from build123d import *

# Parameters (mm, degrees)
STRUCTURAL_MEMBER1_DEPTH = 900
SKETCH12_R               = 4.7625
CUT_EXTRUDE1_DEPTH       = 454.210052427
CUT_EXTRUDE2_DEPTH       = 40
SKETCH16_R               = 4.7625
CUT_EXTRUDE3_DEPTH       = 454.210052526
SKETCH17_R               = 4.7625
CUT_EXTRUDE4_DEPTH       = 454.210052526


with BuildPart() as part:
    # Sketch11 → Structural Member1 (new body)
    with BuildSketch(Plane(origin=(-450, 0, 0), x_dir=(0, 0, -1), z_dir=(1, 0, 0))):
        with BuildLine():
            Line((0, -38.1), (0, 38.1))
            Line((0, 38.1), (38.0492, 38.1))
            Line((38.0492, 38.1), (38.0492, 35.942335136))
            ThreePointArc((38.0492, 35.942335136), (37.447280466, 34.300554363), (35.926803066, 33.436899509))
            Line((35.926803066, 33.436899509), (12.283671721, 29.496090157))
            ThreePointArc((12.283671721, 29.496090157), (8.178382741, 27.164222052), (6.5532, 22.731413966))
            Line((6.5532, 22.731413966), (6.5532, -22.731413966))
            ThreePointArc((6.5532, -22.731413966), (8.178382741, -27.164222052), (12.283671721, -29.496090157))
            Line((12.283671721, -29.496090157), (35.926803066, -33.436899509))
            ThreePointArc((35.926803066, -33.436899509), (37.447280466, -34.300554363), (38.0492, -35.942335136))
            Line((38.0492, -35.942335136), (38.0492, -38.1))
            Line((38.0492, -38.1), (0, -38.1))
        make_face()
    extrude(amount=STRUCTURAL_MEMBER1_DEPTH)

    # Sketch12 → Cut-Extrude1 (cut, through all)
    with BuildSketch(Plane(origin=(0, 0, 0), x_dir=(1, 0, 0), z_dir=(0, 1, 0))):
        with Locations(Location((-425, 20, 0), (0, 0, 270))):
            Circle(SKETCH12_R)
        with Locations(Location((425, 20, 0), (0, 0, 270))):
            Circle(SKETCH12_R)
    extrude(amount=-CUT_EXTRUDE1_DEPTH, mode=Mode.SUBTRACT)

    # Sketch15 → Cut-Extrude2 (cut)
    with BuildSketch(Plane(origin=(0, 0, -6.5532), x_dir=(-1, 0, 0), z_dir=(0, 0, -1))):
        with BuildLine():
            Line((-412.5, -33.1), (-437.5, -33.1))
            ThreePointArc((-437.5, -33.1), (-442.5, -28.1), (-437.5, -23.1))
            Line((-437.5, -23.1), (-412.5, -23.1))
            ThreePointArc((-412.5, -23.1), (-407.5, -28.1), (-412.5, -33.1))
        make_face()
        with BuildLine():
            Line((412.5, -33.1), (437.5, -33.1))
            ThreePointArc((437.5, -33.1), (442.5, -28.1), (437.5, -23.1))
            Line((437.5, -23.1), (412.5, -23.1))
            ThreePointArc((412.5, -23.1), (407.5, -28.1), (412.5, -33.1))
        make_face()
    extrude(amount=CUT_EXTRUDE2_DEPTH, mode=Mode.SUBTRACT)

    # Sketch16 → Cut-Extrude3 (cut, through all)
    with BuildSketch(Plane(origin=(0, 0, 0), x_dir=(1, 0, 0), z_dir=(0, 1, 0))):
        with Locations(Location((-192.7, 20, 0), (0, 0, 270))):
            Circle(SKETCH16_R)
        with Locations(Location((-157.7, 20, 0), (0, 0, 270))):
            Circle(SKETCH16_R)
        with Locations(Location((157.7, 20, 0), (0, 0, 90))):
            Circle(SKETCH16_R)
        with Locations(Location((192.7, 20, 0), (0, 0, 90))):
            Circle(SKETCH16_R)
    extrude(amount=CUT_EXTRUDE3_DEPTH, mode=Mode.SUBTRACT)

    # Sketch17 → Cut-Extrude4 (cut, through all)
    with BuildSketch(Plane.XY):
        with Locations((205.8375, 0.6)):
            Circle(SKETCH17_R)
        with Locations((-205.8375, 0.6)):
            Circle(SKETCH17_R)
    extrude(amount=-CUT_EXTRUDE4_DEPTH, mode=Mode.SUBTRACT)


solid = part.part
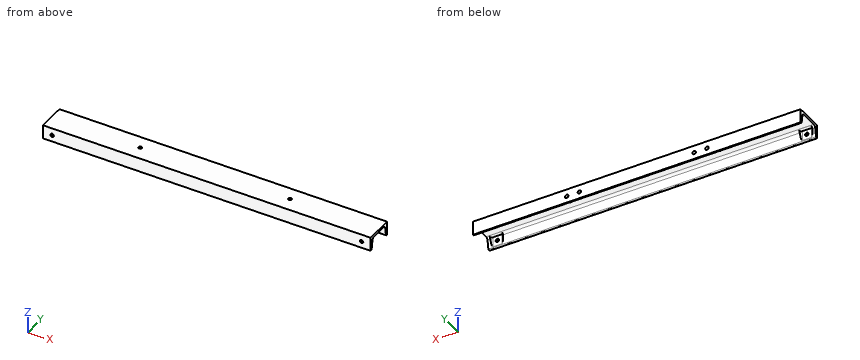
Check sheet for the modelled part. Datum: model origin and axes. Units: mm. Round coordinates to 2 decimals unless told otherwise and drop trailing zeros. Write each loop counter-clockwise with the first axis right and the second up, starting at its lowest first coordinate (ties: lowest second). Pieces come first, ordered by that corner, then holes. Notation, with made-up numbers: (-5.75, 59) - (53.25, 59) arc R27 cw to (53.25, 92) - close; hole circle Ø4 at (39, -30.5). An arc over 180 degrees is marked (long way). Return JSON: item names as keys, results as strings.
Q1. Scan lines: L1, parallel to X at y = 34, z = -20; L2, parallel to X at y = 0, z = -3; L3, parallel to X at y = -34.6, z = -20. Record each from-to range of solid material in increasing order. Write a range as from..to.
Returned:
{"L1": "x = -450..-197.46, -187.94..-162.46, -152.94..152.94, 162.46..187.94, 197.46..450", "L2": "x = -450..-210.56, -201.11..201.11, 210.56..450", "L3": "x = -450..-429.76, -420.24..420.24, 429.76..450"}
Q2. Depth check by flat-ended pin: P1, Ø10, axis at x = 331, y = -1, coming from the -Z side; P2, Ø11, axis at x = 425.5, y = -30, coming from the -Z side; P3, Ø7.5, axis at x = -157.7, z = -20, coming from the +Y side. Enter the tip coordinate at first touch or a pass-through.
Returned:
{"P1": "stops at z = -6.55", "P2": "stops at z = -38.01", "P3": "stops at y = -30.16"}
Q3. Cross-section at A-A (x = 111). Record the boundary of the cut face in (y, z), then the cut area to 3 significant figures.
Returned:
{"outline": "(-38.1, -38.05) - (-35.94, -38.05) arc R2.54 ccw to (-33.44, -35.93) - (-29.5, -12.28) arc R6.86 cw to (-22.73, -6.55) - (22.73, -6.55) arc R6.86 cw to (29.5, -12.28) - (33.44, -35.93) arc R2.54 ccw to (35.94, -38.05) - (38.1, -38.05) - (38.1, 0) - (-38.1, 0) - close", "area": "948 mm²"}
